Can you work these out from the model? Positions are in its coordinate system, mm. A direction names the side the tool comes from. Coordinates: 2 decimals unless noted, no trailing zeros. Write each loop counter-clockwise with the first axis right and the second up, starting at its lowest first coordinate (ties: lowest second). Pieces come first, ordered by that corner, then holes. Notation, with made-up numbers: (65, 18.25) -> (121, 18.25) arc R30 cw to (121, 54.25) -> close; hole circle Ø9 at (62, 75). An arc over 180 degrees is marked (long way). Use one line per item in the form item = value.
```python
from build123d import *

# Parameters (mm, degrees)
F1_DEPTH = 6.35


# Not quite as in the source:
# - ends of sketch curves that miss each other by under 0.0002 mm in the source are joined


with BuildPart() as f1:
    # F0 (on Front) → F1 (new body, symmetric)
    with BuildSketch(Plane.XZ):
        Polygon((-36.8300005794, 19.05), (-43.18, 19.05), (-43.18, -19.05), (43.18, -19.05), (43.18, 19.05), (36.8300005794, 19.05), align=None)
        with BuildLine():
            Line((-43.18, 44.45), (-43.18, 19.05))
            Line((-43.18, 19.05), (-36.8300005794, 19.05))
            Line((-36.8300005794, 19.05), (-36.8300005794, 44.45))
            ThreePointArc((-36.8300005794, 44.45), (0, 81.28), (36.83, 44.45))
            Line((36.83, 44.45), (36.8300005794, 19.05))
            Line((36.8300005794, 19.05), (43.18, 19.05))
            Line((43.18, 19.05), (43.18, 44.45))
            ThreePointArc((43.18, 44.45), (0, 87.63), (-43.18, 44.45))
        make_face()
    extrude(amount=F1_DEPTH, both=True)


solid = f1.part
```
Q1. Thinking about a two-plate mould opening in Z: for faces 1 (the flat face through (-1, 0, -19.05)), 2 (the flat face through (36.83, 0, 32)), 3 (the flat face through (-36.83, 0, 32)), 4 (the flat face through (-43.18, 0, 13)), which applies, released by +Z, released by -Z, zero draft, split by the parting line, or undercut?
Return value:
face_1 = released by -Z
face_2 = undercut
face_3 = undercut
face_4 = zero draft
Q2. Suppose I cut it at B-B (y = 1). Write out the boundary of the cut face in (x, z), then the cut area to 3 significant figures.
Return value:
outline = (-43.18, -19.05) -> (43.18, -19.05) -> (43.18, 44.45) arc R43.18 ccw to (-43.18, 44.45) -> close; hole (-36.83, 19.05) -> (36.83, 19.05) -> (36.83, 44.45) arc R36.83 ccw to (-36.83, 44.45) -> close
area = 4,410 mm2
Q3. Will these pins go through, and if not, where does the flat tip stop? pin 1 (6.5 mm diameter, centred on x = 15, y = -3, fed in from +Z); pin 2 (1 mm diameter, centred on x = -1.5, y = 2.5, fed in from +Z); pin 3 (1 mm diameter, centred on x = 14, y = 0, fed in from +Z).
Return value:
pin_1 = 86
pin_2 = 87.62
pin_3 = 85.47
Q4. Suppose I cut it at C-C (z = 39). Write out the boundary of the cut face in (x, y), then the cut area to 3 significant figures.
Return value:
outline = (-43.18, -6.35) -> (-36.83, -6.35) -> (-36.83, 6.35) -> (-43.18, 6.35) -> close; (36.83, -6.35) -> (43.18, -6.35) -> (43.18, 6.35) -> (36.83, 6.35) -> close
area = 161 mm2
Q5. Suppose I cut it at A-A (x = 0). Write out the boundary of the cut face in (y, z).
Return value:
outline = (-6.35, -19.05) -> (6.35, -19.05) -> (6.35, 19.05) -> (-6.35, 19.05) -> close; (-6.35, 81.28) -> (6.35, 81.28) -> (6.35, 87.63) -> (-6.35, 87.63) -> close
Q6. For faces 5 (the cylindrical face through (-0.81, -0.09, 81.27)), 6 (the flat face through (43.18, 0, 12)), which set-ups out of +Z, -Z, +X, -X, +Y, -Y let a thin tool reach every point of the face, with its end or its side?
Return value:
face_5 = +Y, -Y
face_6 = +Z, -Z, +X, +Y, -Y
Q7. If I drill on line 1 (X direction, y = 2.25, z = 26.5); line 2 (Z direction, x = 1, y = 2.75); line 3 (X direction, y = 0.75, z = 46), over which ranges is the centre line in solid material (lowest first)? Write a range as from..to.
Return value:
line_1 = -43.18..-36.83, 36.83..43.18
line_2 = -19.05..19.05, 81.27..87.62
line_3 = -43.15..-36.8, 36.8..43.15
